from build123d import *

# Parameters (mm, degrees)
F0_W     = 220
F0_H     = 220
F1_DEPTH = 5
F2_R     = 2
F3_DEPTH = 5.001
F4_W     = 20
F4_H     = 120
F4_W_2   = 120
F4_H_2   = 20
F5_DEPTH = 5.001
F6_R     = 10
F7_R     = 4.99999


# Not quite as in the source:
# - a fillet or chamfer is up to 0.001 mm smaller than in the source, because OpenCascade refuses the exact size


with BuildPart() as f1:
    # F0 (on Top) → F1 (new body)
    with BuildSketch(Plane.XY):
        Rectangle(F0_W, F0_H)
    extrude(amount=F1_DEPTH)

    # F2 (on face) → F3 (cut, through all)
    with BuildSketch(Plane.XY.offset(5)):
        with Locations((-97.5, 97.5)):
            Circle(F2_R)
        with Locations((-97.5, -97.5)):
            Circle(F2_R)
        with Locations((97.5, -97.5)):
            Circle(F2_R)
        with Locations((97.5, 97.5)):
            Circle(F2_R)
    extrude(amount=-F3_DEPTH, mode=Mode.SUBTRACT)

    # F4 (on face) → F5 (cut, through all)
    with BuildSketch(Plane(origin=(0, 0, 0), x_dir=(1, 0, 0), z_dir=(0, 0, -1))):
        with Locations((110, 0)):
            Rectangle(F4_W, F4_H)
        with Locations((0, 110)):
            Rectangle(F4_W_2, F4_H_2)
        with Locations((-110, 0)):
            Rectangle(F4_W, F4_H)
        with Locations((0, -110)):
            Rectangle(F4_W_2, F4_H_2)
    extrude(amount=-F5_DEPTH, mode=Mode.SUBTRACT)

    # F6
    f6_edges = [f1.edges().sort_by_distance(p)[0] for p in [
        (110, -110, 2.5),
        (-110, -110, 2.5),
        (110, 110, 2.5),
        (-110, 110, 2.5),
    ]]
    fillet(f6_edges, radius=F6_R)

    # F7 (radius 5 in the source; OpenCascade refuses exactly that, so slightly less here)
    f7_edges = [f1.edges().sort_by_distance(p)[0] for p in [
        (110, 60, 2.5),
        (100, 60, 2.5),
        (100, -60, 2.5),
        (110, -60, 2.5),
        (60, -100, 2.5),
        (60, -110, 2.5),
        (-60, -100, 2.5),
        (-60, -110, 2.5),
        (-100, -60, 2.5),
        (-110, -60, 2.5),
        (-100, 60, 2.5),
        (-110, 60, 2.5),
        (-60, 100, 2.5),
        (-60, 110, 2.5),
        (60, 100, 2.5),
        (60, 110, 2.5),
    ]]
    fillet(f7_edges, radius=F7_R)


solid = f1.part
Could you check a few things on this model? Use its own coordinates, in mm. A direction names the side the tool comes from. Give positions to 0.01 mm unless a question says otherwise; leave off trailing zeros. Order: outer loops, then holes, each group sorted by start corner. A loop starts at its lowest first (then second) coordinate and runs counter-clockwise, first axis right, second up. Notation, with made-up numbers: (26.5, 71) -> (70.5, 71) arc R32 ccw to (70.5, 97) -> close; hole circle Ø9 at (72.25, 24.5). An arc over 180 degrees is marked (long way). Return JSON: item names as keys, results as strings.
1. On a 3-axis mill with a long thin cutter (end or side, diameter ignored), from which of +Z, -Z, +X, -X, +Y, -Y can I reach the whole of each face in a straight line? I mean faces 1 (the flat face through (-1, 100, 2)), 2 (the flat face through (82, 110, 2)), 3 (the cylindrical face through (58, -101, 3)), 4 (the cylindrical face through (-101, 58, 3)), 5 (the cylindrical face through (108, 61, 2)). Say none if no direction works.
Answer list:
{"face 1": "+Z, -Z, +Y", "face 2": "+Z, -Z, +X, -X, +Y", "face 3": "+Z, -Z, -Y", "face 4": "+Z, -Z, -X", "face 5": "+Z, -Z, +X"}
2. Imagine slicing it at B-B on x = -37.5. List the corners of the cut face in (y, z) for me.
Answer list:
{"outline": "(-100, 0) -> (100, 0) -> (100, 5) -> (-100, 5) -> close"}
3. For pin 1 Ø1.5 at (x, z) = (41, 3.5) entering from +Y; pin 2 Ø4.5 at (x, y) = (-97.5, 97.5) entering from -Z; pin 3 Ø2.5 at (x, y) = (97.5, 97.5) entering from +Z; pin 4 Ø2.5 at (x, z) = (-20, 2) entering from -Y, each with a flat end and sliding along its axis, tell me the tip position at first contact or that it passes through.
Answer list:
{"pin 1": "stops at y = 100", "pin 2": "stops at z = 0", "pin 3": "passes through", "pin 4": "stops at y = -100"}
4. I need wall thicknesses on line 1 (Y direction, x = 97.5, z = 3.3); line 2 (Y direction, x = -31, z = 3.75); line 3 (X direction, y = 96, z = 1.8). Which ranges of each line are inside material? Lowest first, please. Write a range as from..to.
Answer list:
{"line 1": "y = -110..-99.5, -95.5..95.5, 99.5..110", "line 2": "y = -100..100", "line 3": "x = -110..-98.82, -96.18..96.18, 98.82..110"}
5. Imagine slicing it at A-A on z = 4.2. Give the number of separate pieces and of enclosed holes in the cut face, then the cut area to 3 significant figures.
Answer list:
{"separate pieces": "1", "enclosed holes": "4", "area": "43,500 mm2"}
